Geometry: final body of the model. Coordinates: model frame, mm. A direction names the side the tool comes from. Coordinates: 2 decimals unless noted, no trailing zeros. Write each loop counter-clockwise with the first axis right and the second up, starting at its lowest first coordinate (ties: lowest second). Pieces come first, ordered by that corner, then holes.
from build123d import *

# Parameters (mm, degrees)
SKETCH4_W                = 18.5
SKETCH4_H                = 32
BOSS_EXTRUDE2_DEPTH      = 2.5
SKETCH5_R                = 16
BOSS_EXTRUDE3_DEPTH      = 2.5
BOSS_EXTRUDE4_DEPTH      = 2.5
BOSS_EXTRUDE4_DEPTH_BACK = 7.5
SKETCH6_W                = 5
SKETCH6_H                = 7
SKETCH9_R                = 2.15
CUT_EXTRUDE1_DEPTH       = 2.5
SKETCH9_3_R              = 3.525
CUT_EXTRUDE3_DEPTH       = 2.5
BOSS_EXTRUDE7_DEPTH      = 10
SKETCH16_W               = 5
SKETCH16_H               = 32
BOSS_EXTRUDE8_DEPTH      = 7.5


with BuildPart() as part:
    # Sketch4 → Boss-Extrude2 (new body)
    with BuildSketch(Plane(origin=(0, 0, 0), x_dir=(1, 0, 0), z_dir=(0, 1, 0))):
        with Locations((11.010130113, -46.927053824)):
            Rectangle(SKETCH4_W, SKETCH4_H)
    extrude(amount=BOSS_EXTRUDE2_DEPTH)

    # Sketch5 → Boss-Extrude3 (add)
    with BuildSketch(Plane(origin=(0, 0, 0), x_dir=(1, 0, 0), z_dir=(0, 1, 0))):
        with Locations((1.760130113, -46.927053824)):
            Circle(SKETCH5_R)
    extrude(amount=BOSS_EXTRUDE3_DEPTH)

    # Sketch6 → Boss-Extrude4 (add, two sides: drawn at the far end of the back side and taken through both)
    with BuildSketch(Plane(origin=(0, 0, 0), x_dir=(1, 0, 0), z_dir=(0, 1, 0)).offset(-BOSS_EXTRUDE4_DEPTH_BACK)):
        with Locations((17.760130113, -66.427053824)):
            Rectangle(SKETCH6_W, SKETCH6_H)
    extrude(amount=BOSS_EXTRUDE4_DEPTH + BOSS_EXTRUDE4_DEPTH_BACK)

    # Sketch9 → Cut-Extrude1 (cut)
    with BuildSketch(Plane(origin=(0, 0, 0), x_dir=(1, 0, 0), z_dir=(0, 1, 0))):
        with Locations(Location((1.760130113, -35.613345325, 0), (0, 0, 270))):
            Circle(SKETCH9_R)
        with Locations(Location((9.760130113, -38.927053824, 0), (0, 0, 270))):
            Circle(SKETCH9_R)
        with Locations(Location((13.073838612, -46.927053824, 0), (0, 0, 270))):
            Circle(SKETCH9_R)
        with Locations(Location((9.760130113, -54.927053824, 0), (0, 0, 270))):
            Circle(SKETCH9_R)
        with Locations(Location((1.760130113, -58.240762323, 0), (0, 0, 270))):
            Circle(SKETCH9_R)
        with Locations(Location((-6.239869887, -54.927053824, 0), (0, 0, 270))):
            Circle(SKETCH9_R)
        with Locations(Location((-9.553578386, -46.927053824, 0), (0, 0, 270))):
            Circle(SKETCH9_R)
        with Locations(Location((-6.239869887, -38.927053824, 0), (0, 0, 270))):
            Circle(SKETCH9_R)
    extrude(amount=CUT_EXTRUDE1_DEPTH, mode=Mode.SUBTRACT)

    # Sketch9_3 → Cut-Extrude3 (cut)
    with BuildSketch(Plane(origin=(0, 0, 0), x_dir=(1, 0, 0), z_dir=(0, 1, 0))):
        with Locations(Location((1.760130113, -46.927053824, 0), (0, 0, 270))):
            Circle(SKETCH9_3_R)
    extrude(amount=CUT_EXTRUDE3_DEPTH, mode=Mode.SUBTRACT)

    # Sketch14 → Boss-Extrude7 (add)
    with BuildSketch(Plane(origin=(0, -7.5, 0), x_dir=(-1, 0, 0), z_dir=(0, -1, 0))):
        with BuildLine():
            Line((-20.260130113, -171.927053824), (-20.260130113, -176.927053824))
            ThreePointArc((-20.260130113, -176.927053824), (-76.260130113, -120.927053824), (-20.260130113, -64.927053824))
            Line((-20.260130113, -64.927053824), (-20.260130113, -69.927053824))
            ThreePointArc((-20.260130113, -69.927053824), (-71.260130113, -120.927053824), (-20.260130113, -171.927053824))
        make_face()
    extrude(amount=-BOSS_EXTRUDE7_DEPTH)

    # Sketch16 → Boss-Extrude8 (add)
    with BuildSketch(Plane(origin=(0, 0, 0), x_dir=(-1, 0, 0), z_dir=(0, -1, 0))):
        with Locations((-17.760130113, -46.927053824)):
            Rectangle(SKETCH16_W, SKETCH16_H)
    extrude(amount=BOSS_EXTRUDE8_DEPTH)


solid = part.part
Item 1: Pin query (flat end, axial travel): pin 1 (6.5 mm diameter, centred on x = 1.76, z = 46.93, fed in from +Y); pin 2 (4 mm diameter, centred on x = 17.5, y = -4.5, fed in from +Z); pin 3 (5.5 mm diameter, centred on x = 1.76, z = 58.24, fed in from -Y); pin 4 (2 mm diameter, centred on x = 10.5, y = 2, fed in from +Z). Return the tip coordinate at first contact, or that it passes through.
Derived:
pin 1: passes through
pin 2: stops at z = 69.93
pin 3: stops at y = 0
pin 4: stops at z = 62.93
Item 2: Pull-direction query (Z, two-part tool) for faces 1 (the flat face through (18, -3, 69.927)), 2 (the flat face through (66, -7.5, 98)), 3 (the cylindrical face through (9.85, 1.23, 52.78)); classes: released by +Z, released by -Z, zero draft, split by the parting line, or undercut.
Derived:
face 1: released by +Z
face 2: zero draft
face 3: undercut
Item 3: Material intervals for probe 1 along X at (y, z) = (-4.5, 39); probe 2 along Z at (x, y) = (61.5, -4.5); probe 3 along Z at (x, y) = (49.5, -7), sorted ascending.
Derived:
probe 1: x = 15.26 to 20.26
probe 2: z = 83.04 to 90.92, 150.93 to 158.81
probe 3: z = 73.17 to 79.14, 162.71 to 168.69
Item 4: Section D-D, the plane z = 89. Output: boundary loops of the cut face in (x, y).
Derived:
outline: (60.03, -7.5) - (66.27, -7.5) - (66.27, 2.5) - (60.03, 2.5) - close
Item 5: Set-up query: faces 4 (the cylindrical face through (76.247, -2.57, 122.158)), 5 (the flat face through (20.26, -3, 174)), 6 (the flat face through (0.3, 0, 50.3)). Return all of +Z, -Z, +X, -X, +Y, -Y with unobstructed straight access to the full face (end or side cutting, diameter ignored); none if empty.
Derived:
face 4: +X, +Y, -Y
face 5: +Z, -X, +Y, -Y
face 6: +Z, -Z, -X, -Y
Item 6: Section A-A, the plane x = 43.5. Output: boundary loops of the cut face in (y, z), plus the area to 3 significant figures.
Derived:
outline: (-7.5, 69.98) - (2.5, 69.98) - (2.5, 75.53) - (-7.5, 75.53) - close; (-7.5, 166.32) - (2.5, 166.32) - (2.5, 171.88) - (-7.5, 171.88) - close
area: 111 mm2
Item 7: Section C-C, the plane x = 56. Output: boundary loops of the cut face in (y, z), plus the area to 3 significant figures.
Derived:
outline: (-7.5, 77.81) - (2.5, 77.81) - (2.5, 84.54) - (-7.5, 84.54) - close; (-7.5, 157.31) - (2.5, 157.31) - (2.5, 164.04) - (-7.5, 164.04) - close
area: 135 mm2
Item 8: Section B-B, the plane y = -4.5. Output: boundary loops of the cut face in (x, z).
Derived:
outline: (15.26, 30.93) - (20.26, 30.93) - (20.26, 64.93) arc R56 ccw to (20.26, 176.93) - (20.26, 171.93) arc R51 cw to (20.26, 69.93) - (15.26, 69.93) - close
